from build123d import *

# Parameters (mm, degrees)
F0_R     = 4.115829
F1_DEPTH = 1.27


with BuildPart() as f1:
    # F0 (on Front) → F1 (new body, symmetric)
    with BuildSketch(Plane.XZ):
        with BuildLine():
            ThreePointArc((-18.938706, 0.359932), (-16.847498, 0.660789), (-14.776399, 0.243397))
            Line((-14.776399, 0.243397), (-14.776399, 30.174541))
            Line((-14.776399, 30.174541), (-18.938706, 30.174541))
            Line((-18.938706, 30.174541), (-18.938706, 0.359932))
        make_face()
        with BuildLine():
            ThreePointArc((-18.938706, 0.359932), (-20.673798, -10.574059), (-10.809144, -5.548992))
            ThreePointArc((-10.809144, -5.548992), (-11.89604, -2.038619), (-14.776399, 0.243397))
            ThreePointArc((-14.776399, 0.243397), (-16.847498, 0.660789), (-18.938706, 0.359932))
        make_face()
        with Locations((-17.021358, -5.548992)):
            Circle(F0_R, mode=Mode.SUBTRACT)
    extrude(amount=F1_DEPTH, both=True)


solid = f1.part
CAD build for the part. Positions are in the model's coordinates, mm. A direction names the side the tool comes from. Give positions to 0.01 mm unless a question says otherwise; leave off trailing zeros. Order: outer loops, then holes, each group sorted by start corner. A loop starts at its lowest first (then second) coordinate and runs counter-clockwise, first axis right, second up. Notation, with made-up numbers: (32.5, -11.75) - (67.5, -11.75) arc R5 ccw to (67.5, -5.75) - close; hole circle Ø3 at (9, 0.5). An arc over 180 degrees is marked (long way). Answer in a Markdown table with one row per item.
1. Pull direction Z, two halves, no side cores. Call faces 3 (the cylindrical face through (-20.29, 0.02, -8.05)), 4 (the flat face through (-17, 0, 30.175)), 5 (the flat face through (-18.939, 0, 15)): pulls with the +Z half, pulls with the -Z half, needs draft (parallel to the pull), parting line crosses it, or undercut.
Data:
| item | result |
|---|---|
| face 3 | undercut |
| face 4 | pulls with the +Z half |
| face 5 | needs draft |
2. Saw through at C-C, the plane y = -0.55. Give the cut face in (x, z).
Data:
| item | result |
|---|---|
| outline | (-18.94, 0.36) arc R6.21 ccw (long way) to (-10.81, -5.55) arc R6.21 ccw to (-14.78, 0.24) - (-14.78, 30.17) - (-18.94, 30.17) - close; hole circle Ø8.23 at (-17.02, -5.55) |
3. Probe probe 1 along Z at (x, y) = (-17.25, 0.8); probe 2 along Z at (x, y) = (-14, 0.35); probe 3 along X at (y, z) = (0.8, -5). List the from-to ranges inside material, lowest first. Write a range as [from, to].
Data:
| item | result |
|---|---|
| probe 1 | z = [-11.76, -9.66], [-1.44, 30.17] |
| probe 2 | z = [-10.98, -8.34], [-2.75, -0.12] |
| probe 3 | x = [-23.21, -21.1], [-12.94, -10.83] |
4. Tool access for faces 1 (the flat face through (-16, -1.27, 9)), 2 (the flat face through (-14.776, 0, 15)): list every direction of +Z, -Z, +X, -X, +Y, -Y with a clear straight run to the whole face (end or side of a thin tool).
Data:
| item | result |
|---|---|
| face 1 | +Z, -Z, +X, -X, -Y |
| face 2 | +Z, +X, +Y, -Y |
5. Flat gauge pins, fed straight in: pin 1 (1.5 mm diameter, centred on x = -14.5, z = 17, fed in from -Y); pin 2 (1 mm diameter, centred on y = 0.5, z = 7, fed in from -X). Where does each tip first touch, or does it go through?
Data:
| item | result |
|---|---|
| pin 1 | stops at y = -1.27 |
| pin 2 | stops at x = -18.94 |
6. Saw through at A-A, the plane x = -14. Give the cut face in (y, z).
Data:
| item | result |
|---|---|
| outline | (-1.27, -10.98) - (1.27, -10.98) - (1.27, -8.34) - (-1.27, -8.34) - close; (-1.27, -2.75) - (1.27, -2.75) - (1.27, -0.12) - (-1.27, -0.12) - close |
7. Saw through at B-B, the plane z = -6.5. Give the cut face in (x, y), plus the area to 3 significant figures.
Data:
| item | result |
|---|---|
| outline | (-23.16, -1.27) - (-21.03, -1.27) - (-21.03, 1.27) - (-23.16, 1.27) - close; (-13.02, -1.27) - (-10.88, -1.27) - (-10.88, 1.27) - (-13.02, 1.27) - close |
| area | 10.8 mm² |
8. Saw through at D-D, the plane z = 17.5. Give the cut face in (x, y).
Data:
| item | result |
|---|---|
| outline | (-18.94, -1.27) - (-14.78, -1.27) - (-14.78, 1.27) - (-18.94, 1.27) - close |
